Part model, mm, in its own coordinate system. Give positions to 0.01 mm unless a question says otherwise; leave off trailing zeros. Loops run counter-clockwise (first coordinate to the right, second up) from the corner with the lowest first, then second, coordinate; pieces in that order, holes last. Notation, with made-up numbers: M 23,62 L 46,62 A19 cw 46,90 Z; hole C -36.75,55 d5. An arc over 180 degrees is marked long. Answer in a Markdown table with one row per item.
from build123d import *

# Parameters (mm, degrees)
F1_DEPTH = 1.27


with BuildPart() as f1:
    # F0 (on Top) → F1 (new body)
    with BuildSketch(Plane.XY):
        with BuildLine():
            Line((-60.090681, -24.242216), (-60.949747, -26.003563))
            Line((-60.949747, -26.003563), (-54.63702, -26.003563))
            ThreePointArc((-54.63702, -26.003563), (-52.960343, -25.371386), (-52.118427, -23.789593))
            Line((-52.118427, -23.789593), (-52.118427, -26.003563))
            Line((-52.118427, -26.003563), (-45.709747, -26.003563))
            Line((-45.709747, -26.003563), (-41.547436, -17.46956))
            Line((-41.547436, -17.46956), (-45.333524, -17.46956))
            Line((-45.333524, -17.46956), (-46.163354, -19.170964))
            Line((-46.163354, -19.170964), (-57.539363, -19.170964))
            ThreePointArc((-57.539363, -19.170964), (-60.07695, -21.610687), (-57.738863, -24.242216))
            Line((-57.738863, -24.242216), (-60.090681, -24.242216))
        make_face()
        with BuildLine():
            Line((-54.63702, -25.610537), (-60.320774, -25.610537))
            Line((-60.320774, -25.610537), (-59.952137, -24.854719))
            Line((-59.952137, -24.854719), (-54.63702, -24.854719))
            ThreePointArc((-54.63702, -24.854719), (-53.246314, -23.464013), (-54.63702, -22.073307))
            Line((-54.63702, -22.073307), (-57.539363, -22.073307))
            Line((-57.539363, -22.073307), (-57.539363, -21.317489))
            Line((-57.539363, -21.317489), (-50.948626, -21.317489))
            Line((-50.948626, -21.317489), (-50.948626, -25.610537))
            Line((-50.948626, -25.610537), (-51.704444, -25.610537))
            Line((-51.704444, -25.610537), (-51.704444, -22.073307))
            Line((-51.704444, -22.073307), (-53.001934, -22.073307))
            ThreePointArc((-53.001934, -22.073307), (-52.688591, -24.364675), (-54.63702, -25.610537))
        make_face(mode=Mode.SUBTRACT)
        Polygon((-49.007684, -25.610537), (-49.763502, -25.610537), (-49.763502, -21.317489), (-45.878878, -21.317489), (-47.972738, -25.610537), (-48.813663, -25.610537), (-47.08844, -22.073307), (-49.007684, -22.073307), align=None, mode=Mode.SUBTRACT)
        Polygon((-45.955337, -25.610537), (-46.796262, -25.610537), (-44.702402, -21.317489), (-43.861477, -21.317489), align=None, mode=Mode.SUBTRACT)
        with BuildLine():
            Line((-54.63702, -23.10122), (-54.63702, -23.857039))
            Line((-54.63702, -23.857039), (-57.539363, -23.857039))
            ThreePointArc((-57.539363, -23.857039), (-59.685887, -21.710514), (-57.539363, -19.56399))
            Line((-57.539363, -19.56399), (-45.917764, -19.56399))
            Line((-45.917764, -19.56399), (-45.087934, -17.862586))
            Line((-45.087934, -17.862586), (-42.176408, -17.862586))
            Line((-42.176408, -17.862586), (-43.344251, -20.257019))
            Line((-43.344251, -20.257019), (-44.185176, -20.257019))
            Line((-44.185176, -20.257019), (-43.38597, -18.618404))
            Line((-43.38597, -18.618404), (-44.615646, -18.618404))
            Line((-44.615646, -18.618404), (-45.445477, -20.319808))
            Line((-45.445477, -20.319808), (-57.539363, -20.319808))
            ThreePointArc((-57.539363, -20.319808), (-58.930069, -21.710514), (-57.539363, -23.10122))
            Line((-57.539363, -23.10122), (-54.63702, -23.10122))
        make_face(mode=Mode.SUBTRACT)
    extrude(amount=F1_DEPTH)


solid = f1.part
(1) Saw through at B-B (x = -49.25). Write the cut outline in (y, z), plus the area to 3 significant figures.
Recorded:
| item | result |
|---|---|
| outline | M -26,0 L -25.61,0 L -25.61,1.27 L -26,1.27 Z; M -21.32,0 L -20.32,0 L -20.32,1.27 L -21.32,1.27 Z; M -19.56,0 L -19.17,0 L -19.17,1.27 L -19.56,1.27 Z |
| area | 2.27 mm^2 |
(2) Pull direction X, two halves, no side cores. Call faces 1 (the face through (-48, -21.317, 1)), 2 (the face through (-52, -23, 0)): +X half, -X half, draft (parallel to the pull), parting line (faces both ways), or undercut.
Recorded:
| item | result |
|---|---|
| face 1 | undercut |
| face 2 | draft |
(3) Saw through at D-D (z = 0.35). Give the number of separate pieces and of enclosed holes in the cut face, plus the area to 3 significant figures.
Recorded:
| item | result |
|---|---|
| separate pieces | 1 |
| enclosed holes | 4 |
| area | 65.4 mm^2 |
(4) Saw through at C-C (y = -21). Write the cut outline in (x, z).
Recorded:
| item | result |
|---|---|
| outline | M -59.98,0 L -59.56,0 L -59.56,1.27 L -59.98,1.27 Z; M -58.73,0 L -43.27,0 L -43.27,1.27 L -58.73,1.27 Z |
(5) Drill centre lines: line 1 along Y through (x, z) = (-52, 0.65); line 2 along Y through (x, z) = (-57.5, 0.85); line 3 along Y through (x, z) = (-47.5, 0.5). Where is each one in solid material? Low to high.
Recorded:
| item | result |
|---|---|
| line 1 | y = -26 to -22.07, -21.32 to -20.32, -19.56 to -19.17 |
| line 2 | y = -26 to -25.61, -24.85 to -23.86, -23.1 to -22.07, -21.32 to -20.32, -19.56 to -19.17 |
| line 3 | y = -26 to -24.64, -22.92 to -22.07, -21.32 to -20.32, -19.56 to -19.17 |
(6) Pin check, flat tip, straight feed: pin 1 Ø0.7 at (x, z) = (-48, 0.5) entering from +Y. Stop position of the tip, or through.
Recorded:
| item | result |
|---|---|
| pin 1 | stops at y = -19.17 |
(7) Saw through at A-A (x = -55.75). Write the cut outline in (y, z), plus the area to 3 significant figures.
Recorded:
| item | result |
|---|---|
| outline | M -26,0 L -25.61,0 L -25.61,1.27 L -26,1.27 Z; M -24.85,0 L -23.86,0 L -23.86,1.27 L -24.85,1.27 Z; M -23.1,0 L -22.07,0 L -22.07,1.27 L -23.1,1.27 Z; M -21.32,0 L -20.32,0 L -20.32,1.27 L -21.32,1.27 Z; M -19.56,0 L -19.17,0 L -19.17,1.27 L -19.56,1.27 Z |
| area | 4.84 mm^2 |
